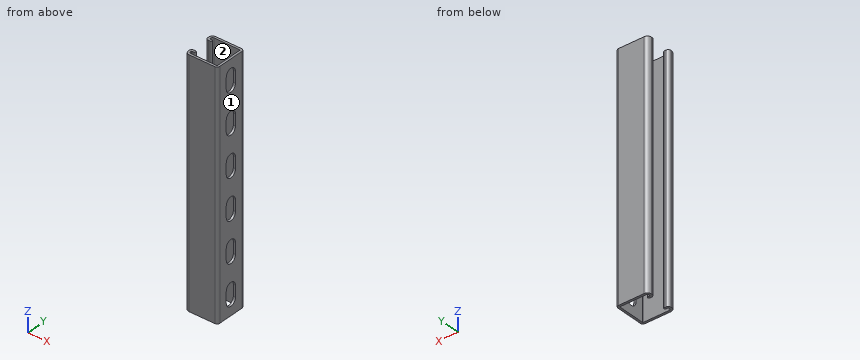
```python
from build123d import *

# Parameters (mm, degrees)
BOSS_EXTRUDE1_DEPTH = 304.8
CUT_EXTRUDE1_DEPTH  = 2.794
LPATTERN1_COUNT     = 6
LPATTERN1_PITCH     = 50.8


with BuildPart() as part:
    # Sketch1 → Boss-Extrude1 (new body)
    with BuildSketch(Plane.XY):
        with BuildLine():
            Line((-36.22675, 20.6375), (-3.46075, 20.6375))
            ThreePointArc((-3.46075, 20.6375), (-1.013630207, 19.623869793), (0, 17.17675))
            Line((0, 17.17675), (0, -17.17675))
            ThreePointArc((0, -17.17675), (-1.013630207, -19.623869793), (-3.46075, -20.6375))
            Line((-3.46075, -20.6375), (-36.22675, -20.6375))
            ThreePointArc((-36.22675, -20.6375), (-39.796401808, -19.158901808), (-41.275, -15.58925))
            Line((-41.275, -15.58925), (-41.275, -14.57325))
            ThreePointArc((-41.275, -14.57325), (-40.261369793, -12.126130207), (-37.81425, -11.1125))
            Line((-37.81425, -11.1125), (-35.5346, -11.1125))
            ThreePointArc((-35.5346, -11.1125), (-34.1376, -12.5095), (-35.5346, -13.9065))
            Line((-35.5346, -13.9065), (-37.81425, -13.9065))
            ThreePointArc((-37.81425, -13.9065), (-38.285713446, -14.101786554), (-38.481, -14.57325))
            Line((-38.481, -14.57325), (-38.481, -15.58925))
            ThreePointArc((-38.481, -15.58925), (-37.820745461, -17.183245461), (-36.22675, -17.8435))
            Line((-36.22675, -17.8435), (-3.46075, -17.8435))
            ThreePointArc((-3.46075, -17.8435), (-2.989286554, -17.648213446), (-2.794, -17.17675))
            Line((-2.794, -17.17675), (-2.794, 17.17675))
            ThreePointArc((-2.794, 17.17675), (-2.989286554, 17.648213446), (-3.46075, 17.8435))
            Line((-3.46075, 17.8435), (-36.22675, 17.8435))
            ThreePointArc((-36.22675, 17.8435), (-37.820745461, 17.183245461), (-38.481, 15.58925))
            Line((-38.481, 15.58925), (-38.481, 14.57325))
            ThreePointArc((-38.481, 14.57325), (-38.285713446, 14.101786554), (-37.81425, 13.9065))
            Line((-37.81425, 13.9065), (-35.5346, 13.9065))
            ThreePointArc((-35.5346, 13.9065), (-34.1376, 12.5095), (-35.5346, 11.1125))
            Line((-35.5346, 11.1125), (-37.81425, 11.1125))
            ThreePointArc((-37.81425, 11.1125), (-40.261369793, 12.126130207), (-41.275, 14.57325))
            Line((-41.275, 14.57325), (-41.275, 15.58925))
            ThreePointArc((-41.275, 15.58925), (-39.796401808, 19.158901808), (-36.22675, 20.6375))
        make_face()
    extrude(amount=-BOSS_EXTRUDE1_DEPTH)

    # Sketch2 → Cut-Extrude1 (cut)
    with BuildSketch(Plane(origin=(0, 0, 0), x_dir=(0, 0, -1), z_dir=(1, 0, 0))):
        with BuildLine():
            Line((18.25625, 7.14375), (32.54375, 7.14375))
            ThreePointArc((32.54375, 7.14375), (39.6875, 0), (32.54375, -7.14375))
            Line((32.54375, -7.14375), (18.25625, -7.14375))
            ThreePointArc((18.25625, -7.14375), (11.1125, 0), (18.25625, 7.14375))
        make_face()
    cut_extrude1 = extrude(amount=-CUT_EXTRUDE1_DEPTH, mode=Mode.SUBTRACT)

    # LPattern1: Cut-Extrude1 ×6
    with Locations(*[(0, 0, -i * LPATTERN1_PITCH) for i in range(1, LPATTERN1_COUNT)]):
        add(cut_extrude1, mode=Mode.SUBTRACT)


solid = part.part
```
Part model, mm, in its own coordinate system. Face numbers are marked on the shaded views. A direction names the side the tool comes from. Round coordinates to 2 decimals unless told otherwise and drop trailing zeros. Write each loop counter-clockwise with the first axis right and the second up, starting at its lowest first coordinate (ties: lowest second). Pieces come first, ordered by that corner, then holes.
Item 1: Cut at C-C, the plane x = -28. Give the cut face in (y, z), plus the area to 3 significant figures.
Results:
outline: (-20.64, -304.8) - (-17.84, -304.8) - (-17.84, 0) - (-20.64, 0) - close; (17.84, -304.8) - (20.64, -304.8) - (20.64, 0) - (17.84, 0) - close
area: 1,700 mm2
Item 2: Which spindle directions (+Z, -Z, +X, -X, +Y, -Y) get a long thin tool onto all of the face, cutting with end or side? Do the marked faces 1 and 2. Say none if no direction does.
Results:
face 1: +Z, -Z, +X, +Y, -Y
face 2: +Z, -Z
Item 3: Drop flat-ended pins along their axis: pin 1 Ø2 at (x, z) = (-1, -181) entering from -Y; pin 2 Ø0.8 at (x, z) = (-1, -226) entering from +Y; pin 3 Ø2 at (x, z) = (-2, -125.5) entering from +Y; pin 4 Ø3 at (x, y) = (-10, 14.5) entering from +Z. Give the stop position or say it passes through.
Results:
pin 1: stops at y = -20.31
pin 2: stops at y = 19.96
pin 3: stops at y = 20.61
pin 4: passes through
Item 4: Probe L1, parallel to Y at x = -36, z = -210; L2, parallel to Y at x = -12, z = -64.5; L3, parallel to X at y = 15, z = -264 (3 decimals). List the from-to ranges inside material, lowest first.
Results:
L1: y = -20.64 to -17.84, -13.91 to -11.11, 11.11 to 13.91, 17.84 to 20.64
L2: y = -20.64 to -17.84, 17.84 to 20.64
L3: x = -41.275 to -38.481, -2.794 to 0
Item 5: Cut at A-A, the plane y = 0. Give the cut face in (x, z), plus the area to 3 significant figures.
Results:
outline: (-2.79, -304.8) - (0, -304.8) - (0, -293.69) - (-2.79, -293.69) - close; (-2.79, -265.11) - (0, -265.11) - (0, -242.89) - (-2.79, -242.89) - close; (-2.79, -214.31) - (0, -214.31) - (0, -192.09) - (-2.79, -192.09) - close; (-2.79, -163.51) - (0, -163.51) - (0, -141.29) - (-2.79, -141.29) - close; (-2.79, -112.71) - (0, -112.71) - (0, -90.49) - (-2.79, -90.49) - close; (-2.79, -61.91) - (0, -61.91) - (0, -39.69) - (-2.79, -39.69) - close; (-2.79, -11.11) - (0, -11.11) - (0, 0) - (-2.79, 0) - close
area: 373 mm2
